The listing builds one solid part. Answer for the finished solid, in the listing's coordinates (mm). A direction names the side the tool comes from. Give positions to 0.01 mm unless a question says otherwise; leave off trailing zeros. Write each loop counter-clockwise with the first axis right and the second up, starting at its lowest first coordinate (ties: lowest second). Pieces come first, ordered by that corner, then holes. Notation, with made-up numbers: (79.5, 11.5) - (131.5, 11.5) arc R24 ccw to (131.5, 31.5) - close; hole circle Ø10 at (51.5, 18). An arc over 180 degrees is marked (long way). One line per question, with ' | ' between items. Start each with the question number.
1. Find the intervals of material crossed by L1, parallel to Y at x = -4.5, z = 0; L2, parallel to X at y = 12.5, z = -10; L3, parallel to X at y = 4, z = -7, in increasing order. Write a range as from..to.
2. For faces 4 (the face through (-0.246, 8.675, -16.679)), 5 (the face through (5.73, -12.4, 2.75)), 6 (the face through (-19.5, -9, 18.1)), determine the directions among +Z, -Z, +X, -X, +Y, -Y from which every point of the face is accessible in a straight line to the end or side of a thin tool.
3. A cutting plane is placed at A-A (x = -10). Determine the outline of the cut face in (y, z), then the cut area to 3 significant figures.
4. A cutting plane is placed at B-B (x = -17). Determine the outline of the cut face in (y, z).
5. Given P1, Ø4, axis at x = -33.5, y = -16.5, coming from the +Z side (3 decimals); P2, Ø5, axis at y = 5, z = 5.5, coming from the -X side; P3, Ø1.5, axis at y = 12, z = 11.5, coming from the +X side, each flat-ended and moving along its own axis, determine where each tip first touches the part or whether it passes through.
6. The mould has two halves that part along Z. Classify faces 1 (the face through (-45.246, 6.007, 19.076)), 2 (the face through (-45, 10.5, 16.4)), 3 (the face through (-7.148, 14.334, 9.139)): +Z half, -Z half, draft (parallel to the pull), parting line (faces both ways), or undercut.
```python
from build123d import *

# Parameters (mm, degrees)
SKETCH1_R           = 19.5
SKETCH1_R_2         = 7.5
BOSS_EXTRUDE1_DEPTH = 4
SKETCH2_R           = 19.5
SKETCH2_R_2         = 17
BOSS_EXTRUDE2_DEPTH = 11.5
SKETCH3_W           = 0.5
SKETCH3_H           = 0.7
SKETCH4_R           = 20.5
SKETCH4_R_2         = 17
BOSS_EXTRUDE3_DEPTH = 8
SKETCH5_R           = 20
SKETCH5_R_2         = 17
BOSS_EXTRUDE4_DEPTH = 28
SKETCH6_W           = 0.5
SKETCH6_H           = 0.7
SKETCH7_R           = 12.7
SKETCH7_R_2         = 7.5
BOSS_EXTRUDE5_DEPTH = 3.5
SKETCH8_R           = 20.5
SKETCH8_R_2         = 3
BOSS_EXTRUDE6_DEPTH = 5


with BuildPart() as part:
    # Sketch1 → Boss-Extrude1 (new body)
    with BuildSketch(Plane(origin=(0, 0, 0), x_dir=(0, 0, -1), z_dir=(1, 0, 0))):
        Circle(SKETCH1_R)
        Circle(SKETCH1_R_2, mode=Mode.SUBTRACT)
    extrude(amount=BOSS_EXTRUDE1_DEPTH)

    # Sketch2 → Boss-Extrude2 (add)
    with BuildSketch(Plane.ZY):
        Circle(SKETCH2_R)
        Circle(SKETCH2_R_2, mode=Mode.SUBTRACT)
    extrude(amount=BOSS_EXTRUDE2_DEPTH)

    # Sketch3 → Cut-Revolve1 (revolve, cut)
    with BuildSketch(Plane.XY):
        with Locations((-0.25, 19.15)):
            Rectangle(SKETCH3_W, SKETCH3_H)
    revolve(axis=Axis((-11.5, 0, 0), (1, 0, 0)), mode=Mode.SUBTRACT)

    # Sketch4 → Boss-Extrude3 (add)
    with BuildSketch(Plane.ZY.offset(11.5)):
        Circle(SKETCH4_R)
        Circle(SKETCH4_R_2, mode=Mode.SUBTRACT)
    extrude(amount=BOSS_EXTRUDE3_DEPTH)

    # Sketch5 → Boss-Extrude4 (add)
    with BuildSketch(Plane.ZY.offset(19.5)):
        Circle(SKETCH5_R)
        Circle(SKETCH5_R_2, mode=Mode.SUBTRACT)
    extrude(amount=BOSS_EXTRUDE4_DEPTH)

    # Sketch6 → Cut-Revolve2 (revolve, cut)
    with BuildSketch(Plane.XY):
        Polygon((-45.5, 20), (-46.5, 20), (-46.15, 19.15), (-45.85, 19.15), align=None)
        with Locations((-44.75, 19.65)):
            Rectangle(SKETCH6_W, SKETCH6_H)
    revolve(axis=Axis((-11.5, 0, 0), (1, 0, 0)), mode=Mode.SUBTRACT)

    # Sketch7 → Boss-Extrude5 (add)
    with BuildSketch(Plane(origin=(4, 0, 0), x_dir=(0, 0, -1), z_dir=(1, 0, 0))):
        Circle(SKETCH7_R)
        Circle(SKETCH7_R_2, mode=Mode.SUBTRACT)
    extrude(amount=BOSS_EXTRUDE5_DEPTH)

    # Sketch8 → Boss-Extrude6 (add)
    with BuildSketch(Plane.ZY.offset(19.5)):
        Circle(SKETCH8_R)
        Circle(SKETCH8_R_2, mode=Mode.SUBTRACT)
    extrude(amount=-BOSS_EXTRUDE6_DEPTH)


solid = part.part
```
Determined:
1) L1: -19.5..-17, 17..19.5 | L2: -19.5..-14.5, 0..4 | L3: -19.5..-14.5, 0..7.5
2) face 4: none | face 5: +X | face 6: -X
3) outline: circle Ø39 at (0, 0); hole circle Ø34 at (0, 0) | area: 287 mm2
4) outline: circle Ø41 at (0, 0); hole circle Ø6 at (0, 0)
5) P1: z = 13.775 | P2: x = -19.5 | P3: x = 4
6) face 1: parting line | face 2: draft | face 3: undercut
